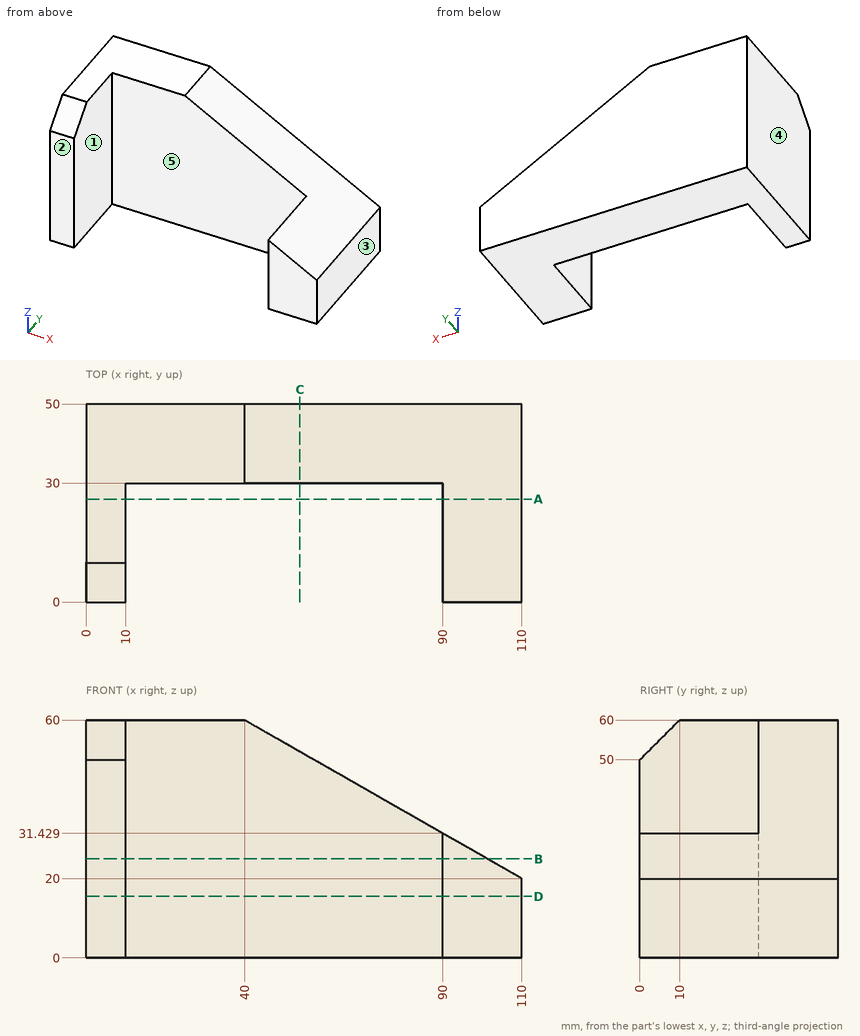
The figure shows three views and two pictorial views of one solid part (mm, origin at its lowest corner). Answer the questions. A direction names the side the tool comes from. Round coordinates to 2 decimals unless told otherwise and drop trailing zeros. Write each loop counter-clockwise with the first axis right and the second up, starting at its lowest first coordinate (ties: lowest second). Pieces come first, ordered by that corner, then holes. Notation, with made-up numbers: (-33.75, -27) -> (-3.75, -27) arc R16 cw to (-3.75, -21) -> close; hole circle Ø5 at (-30, 65.5). An arc over 180 degrees is marked (long way). Answer as a JSON object with one key per item and string values. Group by question number.
Q1. Section A-A (y = 26) is taken. Write down the section's boundary in (x, z).
Q2. Section B-B (z = 25) is taken. Write down the section's boundary in (x, y).
Q3. Determine the mould class of the marked faces 1, 2 and 3 for opening direction X: pulls with the +X half, pulls with the -X half, needs draft (parallel to the pull), parting line crosses it, or undercut.
Q4. Section D-D (z = 15.5) is taken. Write down the section's boundary in (x, y), plus the area to 3 significant figures.
Q5. Each of these flat-tipped pins is pushed along its axis until it touches: pin 1 Ø10 at (x, y) = (81, 8) entering from -Z; pin 2 Ø15 at (y, z) = (8, 20.5) entering from -X; pin 3 Ø1 at (x, y) = (60.5, 37) entering from +Z; pin 4 Ø8 at (x, y) = (70.5, 27.5) entering from +Z (1 decimal). Where does it stop, or does it pass through?
Q6. Which of the six approach directions +Z, -Z, +X, -X, +Y, -Y give full straight-line access (tool end or side, diameter ignored) to the marked faces 4 and 5?
Q7. Straight lines are drawn through the part: line 1 along X through (y, z) = (13.5, 18.5); line 2 along Y through (x, z) = (77, 19); line 3 along X through (y, z) = (10, 49). For each, find the intervals that lie inside material, in ascending order.
Q8. Section C-C (x = 54) is taken. Write down the section's boundary in (y, z).
Check values:
{
 "1": {"outline": "(0, 0) -> (10, 0) -> (10, 60) -> (0, 60) -> close; (90, 0) -> (110, 0) -> (110, 20) -> (90, 31.43) -> close"},
 "2": {"outline": "(0, 0) -> (10, 0) -> (10, 30) -> (90, 30) -> (90, 0) -> (101.25, 0) -> (101.25, 50) -> (0, 50) -> close"},
 "3": {"face 1": "undercut", "face 2": "needs draft", "face 3": "pulls with the +X half"},
 "4": {"outline": "(0, 0) -> (10, 0) -> (10, 30) -> (90, 30) -> (90, 0) -> (110, 0) -> (110, 50) -> (0, 50) -> close", "area": "3,100 mm^2"},
 "5": {"pin 1": "through", "pin 2": "x = 0", "pin 3": "z = 48.57", "pin 4": "z = 44.4"},
 "6": {"face 4": "+Z, -Z, -X, +Y, -Y", "face 5": "+Z, -Z, -Y"},
 "7": {"line 1": "0 to 10, 90 to 110", "line 2": "30 to 50", "line 3": "0 to 10"},
 "8": {"outline": "(30, 0) -> (50, 0) -> (50, 52) -> (30, 52) -> close"}
}
